Can you work these out from the model? Positions are in its coordinate system, mm. A direction names the side the tool comes from. Round coordinates to 2 decimals unless told otherwise and drop trailing zeros. Loops run counter-clockwise (first coordinate to the right, second up) from the corner with the lowest first, then second, coordinate; pieces in that order, holes last.
(1) Will these pins go through, and if not, where does the flat tip stop? pin 1 Ø1.5 at (x, z) = (-10, -37.5) entering from +Y; pin 2 Ø10.5 at (x, y) = (-70, 108) entering from +Z; pin 3 Ø2 at (y, z) = (29, -11.5) entering from -X.
(2) I want a section at D-D on x = -29. Write out the boundary of the cut face in (y, z).
(3) I want a section at B-B on z = -41.5. Write out the boundary of the cut face in (x, y).
(4) Which directions (+Z, -Z, +X, -X, +Y, -Y) give clear straight access to the entire face, cutting with the end or side of a thin tool? Please do faces 1 (the face through (-49, 50, -68)), 2 (the face through (-46, 49, -17)).
(5) I want a section at A-A on x = -63.5. Write out the boundary of the cut face in (y, z), plus the area to 3 significant figures.
(6) If I drill on line 1 along Z through (x, y) = (-29.5, 72); line 2 along Z through (x, y) = (-58.5, 49.5); line 3 along X through (y, z) = (41, -42.5), over which ranges is the centre line in solid material (lowest first)?
(7) I want a section at C-C on y = 67.5. Write out the boundary of the cut face in (x, z).
from build123d import *

# Parameters (mm, degrees)
EXTRUDE1_DEPTH     = 90
CUT_EXTRUDE1_DEPTH = 69
SKETCH4_W          = 158.762085971
SKETCH4_H          = 101.139551932
CUT_EXTRUDE2_DEPTH = 30
EXTRUDE2_DEPTH     = 100
CUT_EXTRUDE3_DEPTH = 69
SKETCH8_W          = 142.373577685
SKETCH8_H          = 89.670115664
CUT_EXTRUDE4_DEPTH = 20
EXTRUDE3_DEPTH     = 120
CUT_EXTRUDE5_DEPTH = 69
SKETCH12_W         = 148.763155866
SKETCH12_H         = 89.075175212
CUT_EXTRUDE6_DEPTH = 20
EXTRUDE4_DEPTH     = 140
CUT_EXTRUDE7_DEPTH = 69
SKETCH16_W         = 108.093048797
SKETCH16_H         = 52.640689948
CUT_EXTRUDE8_DEPTH = 10


with BuildPart() as part:
    # Sketch1 → Extrude1 (new body)
    with BuildSketch(Plane(origin=(0, 0, 0), x_dir=(1, 0, 0), z_dir=(0, 1, 0))):
        Polygon((0, 0), (18.220545085, 68), (-93.220545085, 68), (-75, 0), align=None)
    extrude(amount=EXTRUDE1_DEPTH)

    # Sketch2 → Cut-Extrude1 (cut, through all)
    with BuildSketch(Plane(origin=(0, 0, -68), x_dir=(-1, 0, 0), z_dir=(0, 0, -1))):
        Polygon((-18.220545085, 40), (93.220545085, 80.561239696), (93.220545085, 90), (-18.220545085, 90), align=None)
    extrude(amount=-CUT_EXTRUDE1_DEPTH, mode=Mode.SUBTRACT)

    # Sketch4 → Cut-Extrude2 (cut)
    with BuildSketch(Plane(origin=(4.679123258, 12.855785494, 5.602047686), x_dir=(-0.948588376, 0.290160149, 0.126440426), z_dir=(0.316512391, 0.869610646, 0.378942252))):
        with Locations((41.583207075, -49.139243179)):
            Rectangle(SKETCH4_W, SKETCH4_H)
    extrude(amount=CUT_EXTRUDE2_DEPTH, mode=Mode.SUBTRACT)

    # Sketch5 → Extrude2 (add)
    with BuildSketch(Plane(origin=(0, 0, 0), x_dir=(1, 0, 0), z_dir=(0, 1, 0))):
        Polygon((0.620850018, 68), (-13.044558796, 17), (-79.555136271, 17), (-93.220545085, 68), align=None)
    extrude(amount=EXTRUDE2_DEPTH)

    # Sketch6 → Cut-Extrude3 (cut, through all)
    with BuildSketch(Plane(origin=(0, 0, -68), x_dir=(-1, 0, 0), z_dir=(0, 0, -1))):
        Polygon((-0.620850018, 63.405765137), (93.220545085, 97.561239696), (93.220545085, 100), (-0.620850018, 100), align=None)
    extrude(amount=-CUT_EXTRUDE3_DEPTH, mode=Mode.SUBTRACT)

    # Sketch8 → Cut-Extrude4 (cut)
    with BuildSketch(Plane(origin=(9.358246516, 25.711570987, 11.204095371), x_dir=(-0.948588376, 0.290160149, 0.126440426), z_dir=(0.316512391, 0.869610646, 0.378942252))):
        with Locations((46.415862332, -66.070937723)):
            Rectangle(SKETCH8_W, SKETCH8_H)
    extrude(amount=CUT_EXTRUDE4_DEPTH, mode=Mode.SUBTRACT)

    # Sketch9 → Extrude3 (add)
    with BuildSketch(Plane(origin=(0, 0, 0), x_dir=(1, 0, 0), z_dir=(0, 1, 0))):
        Polygon((-16.978845049, 68), (-26.089117591, 34), (-84.110272543, 34), (-93.220545085, 68), align=None)
    extrude(amount=EXTRUDE3_DEPTH)

    # Sketch10 → Cut-Extrude5 (cut, through all)
    with BuildSketch(Plane(origin=(0, 0, -68), x_dir=(-1, 0, 0), z_dir=(0, 0, -1))):
        Polygon((16.978845049, 86.811530273), (93.220545085, 114.561239696), (93.220545085, 120), (16.978845049, 120), align=None)
    extrude(amount=-CUT_EXTRUDE5_DEPTH, mode=Mode.SUBTRACT)

    # Sketch12 → Cut-Extrude6 (cut)
    with BuildSketch(Plane(origin=(14.037369773, 38.567356481, 16.806143057), x_dir=(-0.948588376, 0.290160149, 0.126440426), z_dir=(0.316512391, 0.869610646, 0.378942252))):
        with Locations((45.030500849, -66.338275795)):
            Rectangle(SKETCH12_W, SKETCH12_H)
    extrude(amount=CUT_EXTRUDE6_DEPTH, mode=Mode.SUBTRACT)

    # Sketch13 → Extrude4 (add)
    with BuildSketch(Plane(origin=(0, 0, 0), x_dir=(1, 0, 0), z_dir=(0, 1, 0))):
        Polygon((-93.220545085, 68), (-32.507987755, 68), (-37.599022411, 49), (-88.129510429, 49), align=None)
    extrude(amount=EXTRUDE4_DEPTH)

    # Sketch14 → Cut-Extrude7 (cut, through all)
    with BuildSketch(Plane(origin=(0, 0, -68), x_dir=(-1, 0, 0), z_dir=(0, 0, -1))):
        Polygon((32.507987755, 109.463675982), (93.220545085, 131.561239696), (93.220545085, 140), (32.507987755, 140), align=None)
    extrude(amount=-CUT_EXTRUDE7_DEPTH, mode=Mode.SUBTRACT)

    # Sketch16 → Cut-Extrude8 (cut)
    with BuildSketch(Plane(origin=(18.716493031, 51.423141974, 22.408190743), x_dir=(-0.948588376, 0.290160149, 0.126440426), z_dir=(0.316512391, 0.869610646, 0.378942252))):
        with Locations((79.37385231, -93.938274555)):
            Rectangle(SKETCH16_W, SKETCH16_H)
    extrude(amount=CUT_EXTRUDE8_DEPTH, mode=Mode.SUBTRACT)


solid = part.part
Filled sheet:
1. pin 1: stops at y = 54.41
1. pin 2: stops at z = -49
1. pin 3: stops at x = -78.35
2. outline: (0, -68) - (91.19, -68) - (76.37, -34) - (59.37, -34) - (51.96, -17) - (34.96, -17) - (27.56, 0) - (0, 0) - close
3. outline: (-86.12, 0) - (11.12, 0) - (11.12, 31.04) - (-6.48, 37.44) - (-6.48, 54.44) - (-24.08, 60.85) - (-24.08, 77.85) - (-86.12, 100.43) - close
4. face 1: -Z, +X, -X, +Y, -Y
4. face 2: +Z, +X, +Y
5. outline: (0, -68) - (120.74, -68) - (112.46, -49) - (95.46, -49) - (88.93, -34) - (71.93, -34) - (64.52, -17) - (47.52, -17) - (40.11, 0) - (0, 0) - close
5. area: 5,500 mm2
6. line 1: z = -68 to -34
6. line 2: z = -68 to -17
6. line 3: x = -86.39 to -6.21
7. outline: (-93.22, -68) - (-10.63, -68) - (-18.81, -61.17) - (-26.09, -34) - (-51.33, -34) - (-71.69, -17) - (-79.56, -17) - close
